Study the drawing (mm; zero at the part's minimum x, y, z) and answer. Give positions to 0.01 mm unless a question says otherwise; leave off trailing zeros. Loops run counter-clockwise (first coordinate to the right, second up) from the corner with the lowest first, then second, coordinate; pieces in that order, holes last. Notation, with made-up numbers: M -33,-7.5 L 0,-7.5 A16 ccw 0,9.5 Z; hole C -29,-16 d3. An arc over 180 degrees is marked long. Use one line per item in the form item = value. Start each with the question number.
1. Straight lines are drawn through the part: line 1 (Y direction, x = 5, z = 0.5); line 2 (Y direction, x = 4, z = 1). For each, find the intervals that lie inside material, in ascending order. Write a range as from..to.
2. The part is cut by section A-A (x = 74). Write down the section's boundary in (y, z).
3. Each of these flat-tipped pins is pushed along its axis until it touches: pin 1 Ø4 at (x, y) = (5, 75) entering from +Z; pin 2 Ø7 at (x, y) = (75, 5) entering from -Z. Where does it stop, or does it pass through?
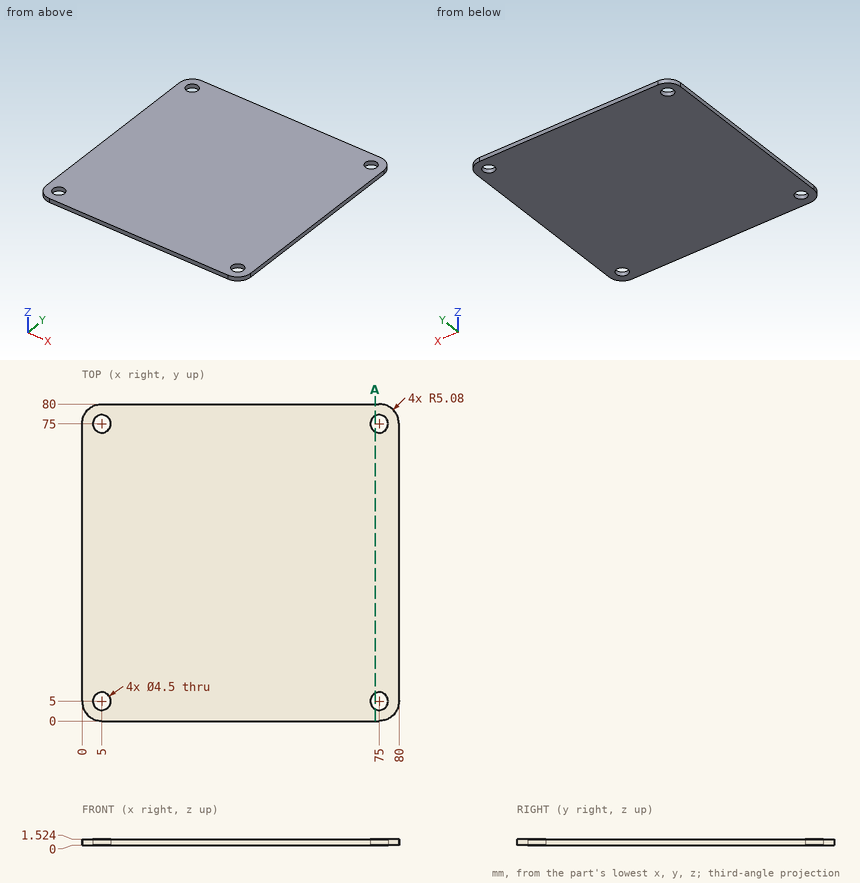
Derived:
q1.line_1 = 0..2.75, 7.25..72.75, 77.25..80
q1.line_2 = 0.12..2.98, 7.02..72.98, 77.02..79.88
q2.outline = M 0,0 L 2.98,0 L 2.98,1.52 L 0,1.52 Z; M 7.02,0 L 72.98,0 L 72.98,1.52 L 7.02,1.52 Z; M 77.02,0 L 80,0 L 80,1.52 L 77.02,1.52 Z
q3.pin_1 = through
q3.pin_2 = 0
